```python
from build123d import *

# Parameters (mm, degrees)
SKETCH2_W           = 81.28
SKETCH2_H           = 55.88
SKETCH2_W_2         = 76.2
SKETCH2_H_2         = 50.8
BOSS_EXTRUDE1_DEPTH = 28.575
SKETCH3_W           = 81.28
SKETCH3_H           = 55.88
BOSS_EXTRUDE2_DEPTH = 2.54
SKETCH6_R           = 2.54
CUT_EXTRUDE2_DEPTH  = 2.54
CHAMFER2_SIZE2      = 1.052102448
CHAMFER2_SIZE       = 2.54
SKETCH7_R           = 12.7
CUT_EXTRUDE5_DEPTH  = 2.54
BOSS_EXTRUDE3_DEPTH = 2.54
CHAMFER3_SIZE       = 2.54
FILLET2_R           = 0.762
FILLET3_R           = 2.54


with BuildPart() as part:
    # Sketch2 → Boss-Extrude1 (new body)
    with BuildSketch(Plane.XY):
        with Locations((-0.567961126, 5.010592309)):
            Rectangle(SKETCH2_W, SKETCH2_H)
        with Locations((-0.567961126, 5.010592309)):
            Rectangle(SKETCH2_W_2, SKETCH2_H_2, mode=Mode.SUBTRACT)
    extrude(amount=-BOSS_EXTRUDE1_DEPTH)

    # Sketch3 → Boss-Extrude2 (add)
    with BuildSketch(Plane(origin=(0, 0, -28.575), x_dir=(-1, 0, 0), z_dir=(0, 0, -1))):
        with Locations((0.567961126, 5.010592309)):
            Rectangle(SKETCH3_W, SKETCH3_H)
    extrude(amount=BOSS_EXTRUDE2_DEPTH)

    # Sketch6 → Cut-Extrude2 (cut)
    with BuildSketch(Plane.ZY.offset(41.207961126)):
        with Locations((-4.445, 1.200592309)):
            Circle(SKETCH6_R)
    extrude(amount=-CUT_EXTRUDE2_DEPTH, mode=Mode.SUBTRACT)

    # Chamfer2
    chamfer2_edges = [part.edges().sort_by_distance(p)[0] for p in [
        (-38.667961126, 1.200592309, -6.985),
    ]]
    chamfer2_side = [part.faces().sort_by_distance(p)[0] for p in [
        (-38.689003175, 1.200592309, -6.985),
    ]]
    chamfer(chamfer2_edges, length=CHAMFER2_SIZE - 0.0001, length2=CHAMFER2_SIZE2 - 0.0001, reference=chamfer2_side[0])  # a hair under: the kernel refuses the full size

    # Sketch7 → Cut-Extrude5 (cut)
    with BuildSketch(Plane(origin=(0, 32.950592309, 0), x_dir=(1, 0, 0), z_dir=(0, 1, 0))):
        with Locations((-0.567961126, -3.175)):
            Circle(SKETCH7_R)
    extrude(amount=-CUT_EXTRUDE5_DEPTH, mode=Mode.SUBTRACT)

    # Sketch8 → Boss-Extrude3 (add)
    with BuildSketch(Plane.XY):
        Polygon((-38.667961126, 30.410592309), (-19.617961126, 30.410592309), (-19.617961126, 31.426592309), (-39.683961126, 31.426592309), (-39.683961126, -21.405407691), (38.548038874, -21.405407691), (38.548038874, 31.426592309), (18.482038874, 31.426592309), (18.482038874, 30.410592309), (37.532038874, 30.410592309), (37.532038874, -20.389407691), (-38.667961126, -20.389407691), align=None)
    extrude(amount=BOSS_EXTRUDE3_DEPTH)

    # Chamfer3
    chamfer3_edges = [part.edges().sort_by_distance(p)[0] for p in [
        (-0.567961126, 30.410592309, -9.525),
    ]]
    chamfer(chamfer3_edges, length=CHAMFER3_SIZE - 0.0001)  # a hair under: the kernel refuses the full size

    # Fillet2
    fillet2_edges = [part.edges().sort_by_distance(p)[0] for p in [
        (-29.650961126, 31.426592309, 0),
        (-39.683961126, 5.010592309, 0),
        (-0.567961126, -21.405407691, 0),
        (38.548038874, 5.010592309, 0),
        (28.515038874, 31.426592309, 0),
    ]]
    fillet(fillet2_edges, radius=FILLET2_R)

    # Fillet3
    fillet3_edges = [part.edges().sort_by_distance(p)[0] for p in [
        (40.072038874, 5.010592309, -31.115),
        (-0.567961126, -22.929407691, -31.115),
        (-41.207961126, 5.010592309, -31.115),
        (-0.567961126, 32.950592309, -31.115),
    ]]
    fillet(fillet3_edges, radius=FILLET3_R)


solid = part.part
```
Check sheet for the modelled part. Datum: model origin and axes. Units: mm. A direction names the side the tool comes from. Give positions to 0.01 mm unless a question says otherwise; leave off trailing zeros. Order: outer loops, then holes, each group sorted by start corner. A loop starts at its lowest first (then second) coordinate and runs counter-clockwise, first axis right, second up. Notation, with made-up numbers: M 0.25,-33 L 52.25,-33 A16 cw 52.25,-19 Z; hole C 77,-13 d3. An arc over 180 degrees is marked long. Answer in a Markdown table with one row per item.
1) Access from +Z, -Z, +X, -X, +Y, -Y to the whole of each face (thin tool, end or side, straight path). Record for faces 1 (the flat face through (-19.618, 31, 1)), 2 (the flat face through (-39.684, 5, 2)), 3 (the flat face through (37.532, 5, -13)), 4 (the flat face through (29, 31.427, 2)).
Filled sheet:
| item | result |
|---|---|
| face 1 | +Z, +Y |
| face 2 | +Z, -X, +Y, -Y |
| face 3 | +Z |
| face 4 | +Z, +X, -X, +Y |
2) Cross-section at A-A, the plane z = -13. Enter the section's corners in (x, y).
Filled sheet:
| item | result |
|---|---|
| outline | M -41.21,-22.93 L 40.07,-22.93 L 40.07,32.95 L -41.21,32.95 Z; hole M -38.67,-20.39 L 37.53,-20.39 L 37.53,30.41 L -38.67,30.41 Z |
3) Gauge pin test, flat ends, axial feed: P1, Ø0.5, axis at y = 31.5, z = 1.5, coming from the -X side; P2, Ø1.4, axis at y = -1.5, z = 2, coming from the +X side; P3, Ø1.4, axis at x = -4, z = 2, coming from the -Y side. Record the tip position at first contact, or that the pin passes through.
Filled sheet:
| item | result |
|---|---|
| P1 | stops at x = -39.68 |
| P2 | stops at x = 38.55 |
| P3 | stops at y = -21.41 |
4) Release check for a two-part mould opening along Z. For faces 5 (the cylindrical face through (-40.444, 5.402, -30.391)), 6 (the flat face through (0, 32.951, -14)), 7 (the conical face through (-41.05, 1.98, -1.96)) record: +Z half, -Z half, draft (parallel to the pull), parting line (faces both ways), or undercut.
Filled sheet:
| item | result |
|---|---|
| face 5 | -Z half |
| face 6 | draft |
| face 7 | undercut |
5) Thickness scan on L1, parallel to Y at x = -13, z = -18.5; L2, parallel to X at y = 25, z = -26.5; L3, parallel to X at y = 7.5, z = 1. Record the ranges inside material, lowest first. Write a range as [from, to].
Filled sheet:
| item | result |
|---|---|
| L1 | y = [-22.93, -20.39], [30.41, 32.95] |
| L2 | x = [-41.21, -38.67], [37.53, 40.07] |
| L3 | x = [-39.68, -38.67], [37.53, 38.55] |
6) Cross-section at B-B, the plane x = -25.5. Enter the section's corners in (y, z) (3 decimals).
Filled sheet:
| item | result |
|---|---|
| outline | M -22.929,-28.575 A2.54 ccw -20.389,-31.115 L 30.411,-31.115 A2.54 ccw 32.951,-28.575 L 32.951,0 L 32.189,0 A0.762 cw 31.427,0.762 L 31.427,2.54 L 30.411,2.54 L 30.411,-28.575 L -20.389,-28.575 L -20.389,2.54 L -21.405,2.54 L -21.405,0.762 A0.762 cw -22.167,0 L -22.929,0 Z |
7) Cross-section at C-C, the plane y = 29.5. Enter the section's corners in (x, z) (3 decimals).
Filled sheet:
| item | result |
|---|---|
| outline | M -41.208,-28.575 A2.54 ccw -38.668,-31.115 L 37.532,-31.115 A2.54 ccw 40.072,-28.575 L 40.072,0 L 39.31,0 A0.762 cw 38.548,0.762 L 38.548,2.54 L 37.532,2.54 L 37.532,-28.575 L -38.668,-28.575 L -38.668,2.54 L -39.684,2.54 L -39.684,0.762 A0.762 cw -40.446,0 L -41.208,0 Z |
